```python
from build123d import *

# Parameters (mm, degrees)
F0_W     = 30
F0_H     = 30
F0_R     = 2.38125
F0_R_2   = 0.79375
F0_R_3   = 3.175
F0_W_2   = 10
F0_H_2   = 10
F0_R_4   = 1.5875
F1_DEPTH = 15
F2_DEPTH = 25


with BuildPart() as f1:
    # F0 (on Top) → F1 (new body)
    with BuildSketch(Plane.XY):
        Rectangle(F0_W, F0_H)
        with Locations((-10, -10)):
            Circle(F0_R, mode=Mode.SUBTRACT)
        with Locations((10, -10)):
            Circle(F0_R_2, mode=Mode.SUBTRACT)
        with Locations((-10, 10)):
            Circle(F0_R_3, mode=Mode.SUBTRACT)
        Rectangle(F0_W_2, F0_H_2, mode=Mode.SUBTRACT)
        with Locations((10, 10)):
            Circle(F0_R_4, mode=Mode.SUBTRACT)
        Rectangle(F0_W_2, F0_H_2)
    extrude(amount=F1_DEPTH)

    # F0 (on Top) → F2 (join)
    with BuildSketch(Plane.XY):
        Rectangle(F0_W_2, F0_H_2)
    extrude(amount=F2_DEPTH)


solid = f1.part
```
Work out the finished part from the listing and answer in its coordinate system (mm). A direction names the side the tool comes from. Give positions to 0.01 mm unless a question says otherwise; leave off trailing zeros. Loops run counter-clockwise (first coordinate to the right, second up) from the corner with the lowest first, then second, coordinate; pieces in that order, holes last. Notation, with made-up numbers: (47.25, 21) -> (74.25, 21) arc R24 cw to (74.25, 59) -> close; hole circle Ø3 at (75.5, 87.25). An arc over 180 degrees is marked (long way). Use CSV: the item, a comma, the result in double quotes.
1. Straight lines are drawn through the part: line 1 (Y direction, x = -10, z = 3.75) (3 decimals); line 2 (Z direction, x = -4, y = 10.25); line 3 (Y direction, x = -11.25, z = 14.5). For each, find the intervals that lie inside material, in ascending order.
Found:
line 1,"-15 to -12.381, -7.619 to 6.825, 13.175 to 15"
line 2,"0 to 15"
line 3,"-15 to -12.03, -7.97 to 7.08, 12.92 to 15"
2. Flat-ended cylindrical pins translate along their axes: pin 1 Ø8 at (y, z) = (-0.5, 20.5) entering from -X; pin 2 Ø3 at (x, z) = (0.5, 22) entering from +Y; pin 3 Ø3 at (y, z) = (0, 22) entering from +X. Find the tip coordinate at first contact, or state that the pin passes through.
Found:
pin 1,"x = -5"
pin 2,"y = 5"
pin 3,"x = 5"
3. The part is cut by section B-B (z = 14.5). State how many separate pieces and enclosed holes the cut face has, then the cut area to 3 significant figures.
Found:
separate pieces,"1"
enclosed holes,"4"
area,"841 mm^2"
4. The part is cut by section D-D (y = -8.5). Write down the section's boundary in (x, z).
Found:
outline,"(-15, 0) -> (-11.85, 0) -> (-11.85, 15) -> (-15, 15) -> close; (-8.15, 0) -> (15, 0) -> (15, 15) -> (-8.15, 15) -> close"
5. A tool of negligible diameter and unlimited length cuts with its end or side. For faces 4 (the flat face through (-5, 0, 20)), 5 (the flat face through (5, 0, 20)), 6 (the flat face through (0, -5, 20)), from which of +Z, -Z, +X, -X, +Y, -Y can it reach the whole face along a straight path? Write none if from no direction.
Found:
face 4,"+Z, -X, +Y, -Y"
face 5,"+Z, +X, +Y, -Y"
face 6,"+Z, +X, -X, -Y"
6. The part is cut by section C-C (x = 10). Write down the section's boundary in (y, z), then the cut area to 3 significant figures.
Found:
outline,"(-15, 0) -> (-10.79, 0) -> (-10.79, 15) -> (-15, 15) -> close; (-9.21, 0) -> (8.41, 0) -> (8.41, 15) -> (-9.21, 15) -> close; (11.59, 0) -> (15, 0) -> (15, 15) -> (11.59, 15) -> close"
area,"379 mm^2"
7. The part is cut by section A-A (y = 10). Write down the section's boundary in (x, z) (1 decimal), then the cut area to 3 significant figures.
Found:
outline,"(-15, 0) -> (-13.2, 0) -> (-13.2, 15) -> (-15, 15) -> close; (-6.8, 0) -> (8.4, 0) -> (8.4, 15) -> (-6.8, 15) -> close; (11.6, 0) -> (15, 0) -> (15, 15) -> (11.6, 15) -> close"
area,"307 mm^2"
8. The mould has two halves that part along Y. Classify faces 1 (the flat face through (0, 0, 0)), 2 (the flat face through (0, 5, 20)), 3 (the cylindrical face through (10.37, -10.7, 7.4)): +Y half, -Y half, draft (parallel to the pull), parting line (faces both ways), or undercut.
Found:
face 1,"draft"
face 2,"+Y half"
face 3,"undercut"
